from build123d import *

# Parameters (mm, degrees)
BOSS_EXTRUDE1_DEPTH = 42.5
SHELL3_START        = -130.355339059
SHELL3_OUTLINE_W    = 56.855339059
SHELL3_OUTLINE_H    = 37.5
SHELL3_DEPTH        = 155.104076401
SHELL3_2_OUTLINE_W  = 4.144660941
SHELL3_2_OUTLINE_H  = 37.5
SHELL3_2_DEPTH      = 15


# Read off the part's stored shape, not the designer's step: Shell3
with BuildPart() as part:
    # Sketch1 → Boss-Extrude1 (new body)
    with BuildSketch(Plane.XY):
        with BuildLine():
            Line((-30, 0), (-50, 0))
            Line((-50, 0), (-106.568542495, 56.568542495))
            ThreePointArc((-106.568542495, 56.568542495), (-117.175144213, 60.961940777), (-127.781745931, 56.568542495))
            Line((-127.781745931, 56.568542495), (-131.317279836, 53.033008589))
            ThreePointArc((-131.317279836, 53.033008589), (-135.710678119, 42.426406871), (-131.317279836, 31.819805153))
            Line((-131.317279836, 31.819805153), (-75.648177206, -23.849297477))
            Line((-75.648177206, -23.849297477), (-50, -35))
            Line((-50, -35), (0, -35))
            Line((0, -35), (0, -30))
            ThreePointArc((0, -30), (-8.786796564, -8.786796564), (-30, 0))
        make_face()
    extrude(amount=BOSS_EXTRUDE1_DEPTH)

    # Shell3 outline → Shell3 (cut)
    with BuildSketch(Plane(origin=(0, 0, 0), x_dir=(0.7071067811865431, 0.707106781186552, 0), z_dir=(0.707106781186552, -0.707106781186543, 0)).offset(SHELL3_START)):
        with Locations((-39.42766953, 21.25)):
            Rectangle(SHELL3_OUTLINE_W, SHELL3_OUTLINE_H)
    extrude(amount=SHELL3_DEPTH, mode=Mode.SUBTRACT)

    # Shell3 2 outline → Shell3 2 (cut)
    with BuildSketch(Plane(origin=(0, 0, 0), x_dir=(0.7071067811865431, 0.707106781186552, 0), z_dir=(0.707106781186552, -0.707106781186543, 0)).offset(SHELL3_START)):
        with Locations((-69.92766953, 21.25)):
            Rectangle(SHELL3_2_OUTLINE_W, SHELL3_2_OUTLINE_H)
    extrude(amount=SHELL3_2_DEPTH, mode=Mode.SUBTRACT)


solid = part.part
Verification items for the finished model (mm, model axes). A direction names the side the tool comes from. Coordinates: 2 decimals unless noted, no trailing zeros. Order: outer loops, then holes, each group sorted by start corner. A loop starts at its lowest first (then second) coordinate and runs counter-clockwise, first axis right, second up. Notation, with made-up numbers: (18, 42) -> (69, 42) arc R12 cw to (69, 60) -> close; hole circle Ø10 at (-27.5, 50). An arc over 180 degrees is marked (long way). Put each result on its own line as item: value. Start each with the question number.
1. Go/stop test with flat-tipped pins: pin 1 Ø10 at (x, z) = (-87.5, 26) entering from -Y; pin 2 Ø5 at (x, z) = (-70.5, 16.5) entering from +Y; pin 3 Ø1.5 at (y, z) = (-0.5, 36) entering from +X. Record where each tip stops, or that it passes through.
2. Cross-section at B-B, the plane y = 39.5. Record the boundary of the cut face in (x, z).
3. Mould release check, pull along Z, two halves, no side actions. Record for faces 3 (the cylindrical face through (-8.555, -9.021, 41.232)), 4 (the flat face through (-99.89, 3.93, 20.99)), 5 (the flat face through (-69, 3, 0)): released by +Z, released by -Z, zero draft, split by the parting line, or undercut.
4. Cross-section at A-A, the plane x = -33. Record the boundary of the cut face in (y, z), then the cut area to 3 significant figures.
5. Cross-section at D-D, the plane y = -6. Record the boundary of the cut face in (x, z), then the cut area to 3 significant figures.
6. Material ranges on L1, parallel to Z at x = -59, y = -24.5; L2, parallel to Y at x = -31.5, z = 41; L3, parallel to X at y = 15, z = 10.5, recorded low to high. Write a range as [from, to].
7. Cross-section at C-C, the plane x = -109.5. Record the boundary of the cut face in (y, z).
8. Access from +Z, -Z, +X, -X, +Y, -Y to the whole of each face (thin tool, end or side, straight path). Record for faces 1 (the flat face through (-72, 4, 2.5)), 2 (the cylindrical face through (-117.01, 60.96, 1.23)).
Computed:
1. pin 1: y = -17
1. pin 2: y = -22.96
1. pin 3: x = -94.71
2. outline: (-135.42, 0) -> (-89.5, 0) -> (-89.5, 2.5) -> (-135.42, 2.5) -> close; (-135.42, 40) -> (-89.5, 40) -> (-89.5, 42.5) -> (-135.42, 42.5) -> close
3. face 3: zero draft
3. face 4: undercut
3. face 5: released by -Z
4. outline: (-35, 0) -> (0, 0) -> (0, 2.5) -> (-35, 2.5) -> close; (-35, 40) -> (0, 40) -> (0, 42.5) -> (-35, 42.5) -> close
4. area: 175 mm2
5. outline: (-93.5, 0) -> (-12, 0) -> (-12, 2.5) -> (-89.96, 2.5) -> (-89.96, 40) -> (-12, 40) -> (-12, 42.5) -> (-93.5, 42.5) -> close
5. area: 540 mm2
6. L1: [0, 2.5], [40, 42.5]
6. L2: [-35, 0]
6. L3: [-114.5, -110.96]
7. outline: (10, 0) -> (58.85, 0) -> (58.85, 2.5) -> (13.54, 2.5) -> (13.54, 40) -> (58.85, 40) -> (58.85, 42.5) -> (10, 42.5) -> close
8. face 1: +X, +Y
8. face 2: +Z, -Z, +Y
